from build123d import *

# Parameters (mm, degrees)
BOSS_EXTRUDE1_DEPTH = 8.128
BOSS_EXTRUDE3_DEPTH = 10.16
FILLET1_R           = 1.5875
SKETCH12_R          = 0.889


with BuildPart() as part:
    # Sketch1 → Boss-Extrude1 (new body)
    with BuildSketch(Plane.XY):
        with BuildLine():
            Line((-243.375083311, 1532.994901352), (-243.375083311, 1536.494901352))
            ThreePointArc((-243.375083311, 1536.494901352), (-241.217924755, 1541.702742796), (-236.010083311, 1543.859901352))
            Line((-236.010083311, 1543.859901352), (-219.510083311, 1543.859901352))
            ThreePointArc((-219.510083311, 1543.859901352), (-214.302241868, 1541.702742796), (-212.145083311, 1536.494901352))
            Line((-212.145083311, 1536.494901352), (-212.145083311, 1532.994901352))
            ThreePointArc((-212.145083311, 1532.994901352), (-214.302241868, 1527.787059909), (-219.510083311, 1525.629901352))
            Line((-219.510083311, 1525.629901352), (-236.010083311, 1525.629901352))
            ThreePointArc((-236.010083311, 1525.629901352), (-241.217924755, 1527.787059909), (-243.375083311, 1532.994901352))
        make_face()
    extrude(amount=BOSS_EXTRUDE1_DEPTH)

    # Sketch3 → Boss-Extrude3 (add)
    with BuildSketch(Plane(origin=(0, 0, 0), x_dir=(-1, 0, 0), z_dir=(0, 0, -1))):
        with BuildLine():
            Line((234.110083311, 1532.363651352), (221.410083311, 1532.363651352))
            ThreePointArc((221.410083311, 1532.363651352), (220.287551296, 1532.828619337), (219.822583311, 1533.951151352))
            Line((219.822583311, 1533.951151352), (219.822583311, 1535.538651352))
            ThreePointArc((219.822583311, 1535.538651352), (220.287551296, 1536.661183368), (221.410083311, 1537.126151352))
            Line((221.410083311, 1537.126151352), (234.110083311, 1537.126151352))
            ThreePointArc((234.110083311, 1537.126151352), (235.232615326, 1536.661183368), (235.697583311, 1535.538651352))
            Line((235.697583311, 1535.538651352), (235.697583311, 1533.951151352))
            ThreePointArc((235.697583311, 1533.951151352), (235.232615326, 1532.828619337), (234.110083311, 1532.363651352))
        make_face()
    extrude(amount=BOSS_EXTRUDE3_DEPTH)

    # Fillet1
    fillet1_edges = [part.edges().sort_by_distance(p)[0] for p in [
        (-220.287551296, 1536.661183368, -10.16),
        (-219.822583311, 1534.744901352, -10.16),
        (-220.287551296, 1532.828619337, -10.16),
        (-227.760083311, 1532.363651352, -10.16),
        (-235.232615326, 1532.828619337, -10.16),
        (-235.697583311, 1534.744901352, -10.16),
        (-235.232615326, 1536.661183368, -10.16),
        (-227.760083311, 1537.126151352, -10.16),
    ]]
    fillet(fillet1_edges, radius=FILLET1_R)

    # Cut-Sweep1: sweep along a path in Sketch13
    with BuildLine(Plane.XY.offset(4.064)) as cut_sweep1_path:
        Line((-243.375083311, 1536.494901352), (-243.375083311, 1532.994901352))
        ThreePointArc((-243.375083311, 1532.994901352), (-241.217924755, 1527.787059909), (-236.010083311, 1525.629901352))
        Line((-236.010083311, 1525.629901352), (-219.510083311, 1525.629901352))
        ThreePointArc((-219.510083311, 1525.629901352), (-214.302241868, 1527.787059909), (-212.145083311, 1532.994901352))
        Line((-212.145083311, 1532.994901352), (-212.145083311, 1536.494901352))
        ThreePointArc((-212.145083311, 1536.494901352), (-214.302241868, 1541.702742796), (-219.510083311, 1543.859901352))
        Line((-219.510083311, 1543.859901352), (-236.010083311, 1543.859901352))
        ThreePointArc((-236.010083311, 1543.859901352), (-241.217924755, 1541.702742796), (-243.375083311, 1536.494901352))
    # Sketch12 → Cut-Sweep1 (sweep, cut)
    with BuildSketch(Plane.ZY.offset(227.760083311)):
        with Locations((4.064, 1543.351901352)):
            Circle(SKETCH12_R)
    sweep(path=cut_sweep1_path.line, mode=Mode.SUBTRACT)


solid = part.part
Can you work these out from the model? Positions are in its coordinate system, mm. A direction names the side the tool comes from. Give positions to 0.01 mm unless a question says otherwise; leave off trailing zeros. Loops run counter-clockwise (first coordinate to the right, second up) from the corner with the lowest first, then second, coordinate; pieces in that order, holes last. Notation, with made-up numbers: M 15.5,61.25 L 60.5,61.25 A12 ccw 60.5,69.25 Z; hole C 48,67.25 d9. An arc over 180 degrees is marked long. One line per item, written item: value. Start each with the question number.
1) If we section it at B-B, the plane x = -232: Write out the boundary of the cut face in (y, z) (1 decimal), and give its area (3 significant figures).
2) If we section it at D-D, the plane z = 1.5: Write out the boundary of the cut face in (x, y) (3 decimals), and give its area (3 significant figures).
3) I'm going to push flat-ended pins straight in: pin 1 (5 mm diameter, centred on x = -239.5, y = 1535, fed in from -Z); pin 2 (0.5 mm diameter, centred on y = 1535, z = -6, fed in from -X); pin 3 (2 mm diameter, centred on x = -212.65, z = 4.06, fed in from +Y). Where does each tip first touch, or does it pass through?
4) If I drill on line 1 (Y direction, x = -226, z = -3.5); line 2 (Z direction, x = -234, y = 1527.75); line 3 (Y direction, x = -239, z = 5.25), over which ranges is the centre line in solid material (lowest first)? Write a range as [from, to].
5) Thinking about a two-plate mould opening in X: for faces 1 (the face through (-212.145, 1535, 2)), 2 (the face through (-228, 1537.126, -4)), 3 (the face through (-227.876, 1542.463, 4.037)), which applies, +X half, -X half, draft (parallel to the pull), parting line (faces both ways), or undercut?
6) If we section it at A-A, the plane z = -4: Write out the boundary of the cut face in (x, y) (1 decimal).
7) On a 3-axis mill with a long thin cutter (end or side, diameter ignored), from which of +Z, -Z, +X, -X, +Y, -Y can I reach the whole of each face in a straight line? I mean faces 4 (the face through (-235.22, 1536.673, -4.226)), 5 (the face through (-219.823, 1535, -4)), 6 (the face through (-214.4, 1541.8, 1.6)), 7 (the face through (-220.275, 1536.649, -4.226)), 8 (the face through (-235.245, 1532.841, -4.226)). Say none if no direction works.
8) If we section it at C-C, the plane y = 1536: Write out the boundary of the cut face in (x, z), and give its area (3 significant figures).
Completed:
1. outline: M 1525.6,0 L 1532.4,0 L 1532.4,-8.6 A1.6 ccw 1534,-10.2 L 1535.5,-10.2 A1.6 ccw 1537.1,-8.6 L 1537.1,0 L 1543.9,0 L 1543.9,3.3 A0.9 cw long 1543.9,4.8 L 1543.9,8.1 L 1525.6,8.1 L 1525.6,4.8 A0.9 cw long 1525.6,3.3 Z
1. area: 191 mm^2
2. outline: M -243.375,1532.995 A7.365 ccw -236.01,1525.63 L -219.51,1525.63 A7.365 ccw -212.145,1532.995 L -212.145,1536.495 A7.365 ccw -219.51,1543.86 L -236.01,1543.86 A7.365 ccw -243.375,1536.495 Z
2. area: 523 mm^2
3. pin 1: stops at z = 0
3. pin 2: stops at x = -235.7
3. pin 3: stops at y = 1540.51
4. line 1: y = [1532.36, 1537.13]
4. line 2: z = [0, 8.13]
4. line 3: y = [1526.26, 1543.23]
5. face 1: +X half
5. face 2: draft
5. face 3: undercut
6. outline: M -235.7,1534 A1.6 ccw -234.1,1532.4 L -221.4,1532.4 A1.6 ccw -219.8,1534 L -219.8,1535.5 A1.6 ccw -221.4,1537.1 L -234.1,1537.1 A1.6 ccw -235.7,1535.5 Z
7. face 4: -Z, -X, +Y
7. face 5: -Z, +X, +Y, -Y
7. face 6: +Z, -Z, +X, +Y
7. face 7: -Z, +X, +Y
7. face 8: -Z, -X, -Y
8. outline: M -243.38,0 L -235.63,0 L -235.63,-8.57 A1.52 ccw -234.11,-10.09 L -221.41,-10.09 A1.52 ccw -219.89,-8.57 L -219.89,0 L -212.15,0 L -212.15,3.33 A0.89 cw long -212.15,4.79 L -212.15,8.13 L -243.38,8.13 L -243.38,4.79 A0.89 cw long -243.38,3.33 Z
8. area: 407 mm^2
